Autodesk Inventor part; units mm, degrees
ref_plane "YZ Plane" through (0, 0, 0) normal (1, 0, 0) x (0, 1, 0)
ref_plane "XZ Plane" through (0, 0, 0) normal (0, 1, 0) x (-1, 0, 0)
ref_plane "XY Plane" through (0, 0, 0) normal (0, 0, 1) x (1, 0, 0)
sketch "Sketch1" plane through (0, 0, 0) normal (0, 0, 1) x (1, 0, 0)
  circle A0 centre (-12.7, 12.7) radius 2.4892
  line L0 (19.05, 0) -> (-44.45, 0)
  line L1 (-44.45, 0) -> (-44.45, -25.4)
  line L2 (-44.45, -25.4) -> (19.05, -25.4)
  line L3 (19.05, -25.4) -> (19.05, 0)
  line L4 (19.05, 0) -> (-44.45, -25.4) construction
  line L5 (-44.45, 0) -> (19.05, -25.4) construction
  line L6 (0, 57.15) -> (-25.4, 57.15)
  line L7 (-25.4, 57.15) -> (-25.4, 0)
  line L8 (-25.4, 0) -> (0, 0)
  line L9 (0, 0) -> (0, 57.15)
  line L10 (0, 57.15) -> (-25.4, 0) construction
  line L11 (-25.4, 57.15) -> (0, 0) construction
  line L12 (-25.4, 57.15) -> (-44.45, 0)
  circle A1 centre (-12.7, 25.4) radius 2.4892
  circle A2 centre (-12.7, 38.1) radius 2.4892
  circle A3 centre (-12.7, 50.8) radius 2.4892
  circle A4 centre (-38.1, -12.7) radius 2.4892
  circle A5 centre (-25.4, -12.7) radius 2.4892
  circle A6 centre (-12.7, -12.7) radius 2.4892
  circle A7 centre (0, -12.7) radius 2.4892
  circle A8 centre (12.7, -12.7) radius 2.4892
  line L13 (0, 57.15) -> (-8.382, 57.15)
  line L14 (-8.382, 57.15) -> (-8.382, 19.05)
  line L15 (-8.382, 19.05) -> (0, 19.05)
  line L16 (0, 19.05) -> (0, 57.15)
  point P0 (0, 0)
  point P1 (-12.7, -12.7)
  point P2 (-12.7, 28.575)
  point P3 (-12.7, 57.15)
  point P4 (-44.45, -12.7)
  point P5 (0, 19.05)
  dimension "d0" = 4.9784
  dimension "d1" = 25.4
  dimension "d2" = 25.4
  dimension "d5" = 12.7
  dimension "d10" = 6.35
  dimension "d11" = 12.7
  dimension "d12" = 19.05
  dimension "d15" = 12.7
  dimension "d21" = 6.35
  dimension "d25" = 8.382
  dimension "d26" = 6.35
  dimension "d28" = 6.35
extrude "Extrusion1" add sketch "Sketch1" along normal blind 3.175 contours L3 L2 L1 L0 | L0 L7 L6 L14 L15 L9 | L0 L12 L7
fillet "Fillet1" radius 3.175 8 edges at (19.05, 0, 1.5875) (19.05, -25.4, 1.5875) (-44.45, -25.4, 1.5875) (0, 0, 1.5875) (-44.45, 0, 1.5875) (-25.4, 57.15, 1.5875) (-8.382, 57.15, 1.5875) (0, 19.05, 1.5875)
fillet "Fillet1" radius 2 1 edges at (-8.382, 19.05, 1.5875)
equation "\"d28\" = d21"
properties part number "Elevator Mounting Gusset" material "Aluminum 6061"
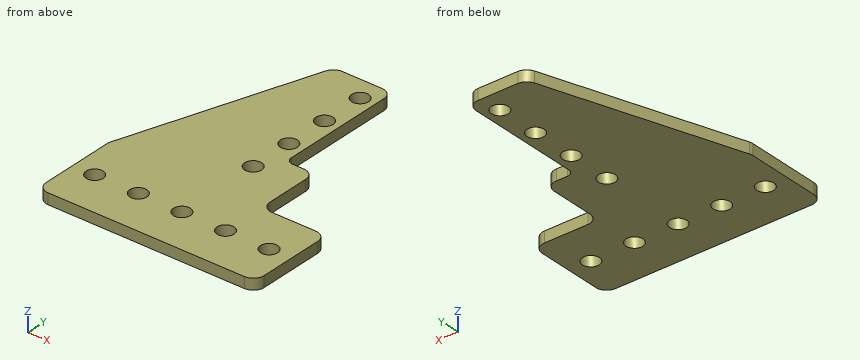
Geometry: final body of the model. Coordinates: model frame, mm. Coordinates: 2 decimals unless noted, no trailing zeros. Order: outer loops, then holes, each group sorted by start corner. A loop starts at its lowest first (then second) coordinate and runs counter-clockwise, first axis right, second up. Notation, with made-up numbers: (-5.75, 84) -> (42.25, 84) arc R16 ccw to (42.25, 105) -> close; hole circle Ø1 at (88, 11). An arc over 180 degrees is marked (long way). Write each question's results on one line, items separated by ' | '. Start each with the question number.
1) Cut plane D-D, the plane z = 2.65. State how many separate pieces and enclosed holes the cut face has, and give its area (3 significant figures).
2) Material intervals for line 1 along Y through (x, z) = (-12.7, 2.45); line 2 along Y through (x, z) = (13, 2.9); line 3 along Y through (x, z) = (16, 1.5), sorted ascending.
3) First-contact query: pin 1 (1 mm diameter, centred on x = 11, z = 2, fed in from +Y); pin 2 (1.6 mm diameter, centred on y = 10, z = 1, fed in from +X). Flat tips, straight axial feed; report the tip coordinate or a pass-through.
4) Cut plane B-B, the plane x = -38.1. Output: boundary loops of the cut face in (y, z) (3 decimals).
5) Cut plane A-A, the plane x = -12.7. Output: boundary loops of the cut face in (y, z) (3 decimals).
6) Cut plane C-C, the plane y = -12.7. Output: boundary loops of the cut face in (x, z) (3 decimals).
Checks:
1) separate pieces: 1 | enclosed holes: 9 | area: 3,110 mm^2
2) line 1: -25.4 to -15.19, -10.21 to 10.21, 15.19 to 22.91, 27.89 to 35.61, 40.59 to 48.31, 53.29 to 57.15 | line 2: -25.4 to -15.17, -10.23 to 0 | line 3: -25.4 to 0
3) pin 1: y = 0 | pin 2: x = 0
4) outline: (-25.4, 0) -> (-15.189, 0) -> (-15.189, 3.175) -> (-25.4, 3.175) -> close; (-10.211, 0) -> (19.05, 0) -> (19.05, 3.175) -> (-10.211, 3.175) -> close
5) outline: (-25.4, 0) -> (-15.189, 0) -> (-15.189, 3.175) -> (-25.4, 3.175) -> close; (-10.211, 0) -> (10.211, 0) -> (10.211, 3.175) -> (-10.211, 3.175) -> close; (15.189, 0) -> (22.911, 0) -> (22.911, 3.175) -> (15.189, 3.175) -> close; (27.889, 0) -> (35.611, 0) -> (35.611, 3.175) -> (27.889, 3.175) -> close; (40.589, 0) -> (48.311, 0) -> (48.311, 3.175) -> (40.589, 3.175) -> close; (53.289, 0) -> (57.15, 0) -> (57.15, 3.175) -> (53.289, 3.175) -> close
6) outline: (-44.45, 0) -> (-40.589, 0) -> (-40.589, 3.175) -> (-44.45, 3.175) -> close; (-35.611, 0) -> (-27.889, 0) -> (-27.889, 3.175) -> (-35.611, 3.175) -> close; (-22.911, 0) -> (-15.189, 0) -> (-15.189, 3.175) -> (-22.911, 3.175) -> close; (-10.211, 0) -> (-2.489, 0) -> (-2.489, 3.175) -> (-10.211, 3.175) -> close; (2.489, 0) -> (10.211, 0) -> (10.211, 3.175) -> (2.489, 3.175) -> close; (15.189, 0) -> (19.05, 0) -> (19.05, 3.175) -> (15.189, 3.175) -> close
